from build123d import *

# Parameters (mm, degrees)
SKETCH1_R           = 14
BOSS_EXTRUDE1_DEPTH = 44
SKETCH2_R           = 9
BOSS_EXTRUDE2_DEPTH = 40
SKETCH3_R           = 5
CUT_EXTRUDE1_DEPTH  = 62.090097558


with BuildPart() as part:
    # Sketch1 → Boss-Extrude1 (new body)
    with BuildSketch(Plane.XY):
        Circle(SKETCH1_R)
    extrude(amount=BOSS_EXTRUDE1_DEPTH)

    # Sketch2 → Boss-Extrude2 (add)
    with BuildSketch(Plane(origin=(0, 0, 0), x_dir=(1, 0, 0), z_dir=(0, 1, 0))):
        with Locations(Location((0, -22, 0), (0, 0, 90))):
            Circle(SKETCH2_R)
    extrude(amount=BOSS_EXTRUDE2_DEPTH)

    # Sketch3 → Cut-Extrude1 (cut, through all)
    with BuildSketch(Plane.XY.offset(44)):
        Circle(SKETCH3_R)
    extrude(amount=-CUT_EXTRUDE1_DEPTH, mode=Mode.SUBTRACT)


solid = part.part
Source: CAD feature listing. Evaluate the final solid. Frame: model axes, mm. A direction names the side the tool comes from. Coordinates: 2 decimals unless noted, no trailing zeros. Order: outer loops, then holes, each group sorted by start corner. A loop starts at its lowest first (then second) coordinate and runs counter-clockwise, first axis right, second up.
Item 1: Set-up query: faces 4 (the face through (0, -6, 0)), 5 (the face through (-2.703, 25.157, 13.416)). Return all of +Z, -Z, +X, -X, +Y, -Y with unobstructed straight access to the full face (end or side cutting, diameter ignored); none if empty.
Output values:
face 4: -Z, +X, -X, +Y, -Y
face 5: +Y
Item 2: Cut plane B-B (y = 0). Return loops of the section in (x, z), plus the area to 3 significant figures.
Output values:
outline: (-14, 0) - (-5, 0) - (-5, 44) - (-14, 44) - close; (5, 0) - (14, 0) - (14, 44) - (5, 44) - close
area: 792 mm2
Item 3: First-contact query: P1, Ø2, axis at y = -6.5, z = 18, coming from the +X side; P2, Ø2, axis at x = 2, z = 39, coming from the +Y side; P3, Ø3, axis at x = 3, z = 23, coming from the -Y side. Flat tips, straight axial feed; report the tip coordinate or a pass-through.
Output values:
P1: stops at x = 12.87
P2: stops at y = 13.96
P3: stops at y = -13.92
Item 4: Pull-direction query (Y, two-part tool) for faces 1 (the face through (-3.03, -13.67, 21.69)), 2 (the face through (0, -6, 44)), 3 (the face through (-1.08, -4.88, 22.31)); classes: pulls with the +Y half, pulls with the -Y half, needs draft (parallel to the pull), parting line crosses it, or undercut.
Output values:
face 1: parting line crosses it
face 2: needs draft
face 3: undercut
Item 5: Material intervals for line 1 (Y direction, x = 0, z = 27); line 2 (Y direction, x = 0, z = 31.5); line 3 (X direction, y = -2, z = 7.5), sorted ascending.
Output values:
line 1: y = -14 to -5, 5 to 40
line 2: y = -14 to -5, 5 to 14
line 3: x = -13.86 to -4.58, 4.58 to 13.86
Item 6: Cut plane C-C (z = 22). Return loops of the section in (x, y), plus the area to 3 significant figures.
Output values:
outline: (-9, 10.72) arc R14 ccw (long way) to (9, 10.72) - (9, 40) - (-9, 40) - close; hole circle Ø10 at (0, 0)
area: 1,020 mm2
Item 7: Cut plane A-A (x = 0). Return loops of the section in (y, z), plus the area to 3 significant figures.
Output values:
outline: (-14, 0) - (-5, 0) - (-5, 44) - (-14, 44) - close; (5, 0) - (14, 0) - (14, 13) - (40, 13) - (40, 31) - (14, 31) - (14, 44) - (5, 44) - close
area: 1,260 mm2
Item 8: Cut plane D-D (x = -8.25). Return loops of the section in (y, z), plus the area to 3 significant figures.
Output values:
outline: (-11.31, 0) - (11.31, 0) - (11.31, 18.4) - (40, 18.4) - (40, 25.6) - (11.31, 25.6) - (11.31, 44) - (-11.31, 44) - close
area: 1,200 mm2
